```python
from build123d import *

# Parameters (mm, degrees)
SZKIC1_W                    = 80
SZKIC1_H                    = 80
DODANIE_WYCI_GNI_CIE1_DEPTH = 60
SZKIC2_W                    = 77
SZKIC2_H                    = 57
WYTNIJ_WYCI_GNI_CIE1_DEPTH  = 108.703296143
SZKIC4_R                    = 4
WYTNIJ_WYCI_GNI_CIE2_DEPTH  = 81.305666052
SZKIC3_R                    = 4
WYTNIJ_WYCI_GNI_CIE3_DEPTH  = 60
ZAOKR_GLENIE1_R             = 5
SFAZOWANIE1_SIZE            = 1


with BuildPart() as part:
    # Szkic1 → Dodanie-wyciągnięcie1 (new body)
    with BuildSketch(Plane(origin=(0, 0, 0), x_dir=(1, 0, 0), z_dir=(0, 1, 0))):
        Rectangle(SZKIC1_W, SZKIC1_H)
    extrude(amount=DODANIE_WYCI_GNI_CIE1_DEPTH)

    # Szkic2 → Wytnij-wyciągnięcie1 (cut, through all)
    with BuildSketch(Plane.XY.offset(40)):
        with Locations((1.5, 31.5)):
            Rectangle(SZKIC2_W, SZKIC2_H)
    extrude(amount=-WYTNIJ_WYCI_GNI_CIE1_DEPTH, mode=Mode.SUBTRACT)

    # Szkic4 → Wytnij-wyciągnięcie2 (cut, through all)
    with BuildSketch(Plane(origin=(0, 3, 0), x_dir=(1, 0, 0), z_dir=(0, 1, 0))):
        with Locations(Location((20, -20, 0), (0, 0, 180))):
            Circle(SZKIC4_R)
        with Locations(Location((20, 20, 0), (0, 0, 180))):
            Circle(SZKIC4_R)
        with Locations(Location((-20, 20, 0), (0, 0, 180))):
            Circle(SZKIC4_R)
        with Locations((-20, -20)):
            Circle(SZKIC4_R)
    extrude(amount=-WYTNIJ_WYCI_GNI_CIE2_DEPTH, mode=Mode.SUBTRACT)

    # Szkic3 → Wytnij-wyciągnięcie3 (cut)
    with BuildSketch(Plane(origin=(-37, 0, 0), x_dir=(0, 0, -1), z_dir=(1, 0, 0))):
        with Locations(Location((-20, 46.5, 0), (0, 0, 90))):
            Circle(SZKIC3_R)
        with Locations((-20, 16.5)):
            Circle(SZKIC3_R)
        with Locations(Location((20, 16.5, 0), (0, 0, 90))):
            Circle(SZKIC3_R)
        with Locations((20, 46.5)):
            Circle(SZKIC3_R)
    extrude(amount=-WYTNIJ_WYCI_GNI_CIE3_DEPTH, mode=Mode.SUBTRACT)

    # Zaokrąglenie1
    zaokr_glenie1_edges = [part.edges().sort_by_distance(p)[0] for p in [
        (-38.5, 60, -40),
        (40, 1.5, 40),
        (40, 1.5, -40),
        (-38.5, 60, 40),
    ]]
    fillet(zaokr_glenie1_edges, radius=ZAOKR_GLENIE1_R)

    # Sfazowanie1
    sfazowanie1_edges = [part.edges().sort_by_distance(p)[0] for p in [
        (-24, 3, 20),
        (-24, 0, 20),
        (-16, 0, -20),
        (-16, 3, -20),
        (24, 3, -20),
        (24, 0, -20),
        (24, 0, 20),
        (24, 3, 20),
        (-40, 46.5, -16),
        (-37, 46.5, -16),
        (-40, 12.5, -20),
        (-37, 12.5, -20),
        (-40, 16.5, 24),
        (-37, 16.5, 24),
        (-40, 42.5, 20),
        (-37, 42.5, 20),
    ]]
    chamfer(sfazowanie1_edges, length=SFAZOWANIE1_SIZE)


solid = part.part
```
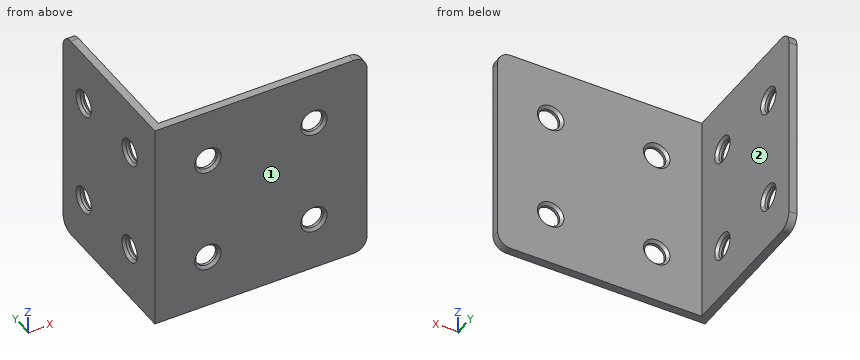
CAD build for the part. Positions are in the model's coordinates, mm. Face numbers are marked on the shaded views. A direction names the side the tool comes from. Give positions to 0.01 mm unless a question says otherwise; leave off trailing zeros. Write each loop counter-clockwise with the first axis right and the second up, starting at its lowest first coordinate (ties: lowest second). Pieces come first, ordered by that corner, then holes. Notation, with made-up numbers: M 17,-5 L 61,-5 A27 cw 61,33 Z; hole C 13.25,14.25 d10. An arc over 180 degrees is marked long. Return JSON: item names as keys, results as strings. Group by question number.
(1) Band-saw the part on C-C (z = 20). State how many separate pieces and enclosed holes the cut face has, and give its area (3 significant figures).
(2) 3-axis set-ups, long thin cutter, end or side, ignore diameter. For the marked faces 1 and 2: which of +Z, -Z, +X, -X, +Y, -Y reach the whole face in a straight line?
(3) Band-saw the part on A-A (x = -20). Give the cut face in (y, z), and give its area (3 significant figures).
(4) Drill centre lines: L1, parallel to Z at x = -20, y = 1.45; L2, parallel to X at y = 14.5, z = -25; L3, parallel to Y at x = -26, z = 31. Where is each one in solid material? Low to high. Write a range as [from, to].
(5) Band-saw the part on B-B (y = 16.5). Give the cut face in (x, z), and give its area (3 significant figures).
(6) Flat gauge pins, fed straight in: pin 1 Ø1.5 at (x, z) = (-4.5, -11.5) entering from +Y; pin 2 Ø10.5 at (y, z) = (46.5, 20) entering from +X. Where does each tip first touch, or does it go through?
(7) Band-saw the part on D-D (z = -6). Give the cut face in (x, y), and give its area (3 significant figures).
Entries:
{
 "1": {"separate pieces": "5", "enclosed holes": "0", "area": "307 mm^2"},
 "2": {"face 1": "+Z, -Z, +X, -X, -Y", "face 2": "+Z, -Z, +X, +Y"},
 "3": {"outline": "M 0,-40 L 3,-40 L 3,-25 L 2,-24 L 1,-24 L 0,-25 Z; M 0,-15 L 1,-16 L 2,-16 L 3,-15 L 3,15 L 2,16 L 1,16 L 0,15 Z; M 0,25 L 1,24 L 2,24 L 3,25 L 3,40 L 0,40 Z", "area": "188 mm^2"},
 "4": {"L1": "z = [-40, -24], [-16, 16], [24, 40]", "L2": "x = [-40, -37]", "L3": "y = [0, 3]"},
 "5": {"outline": "M -40,-40 L -37,-40 L -37,-25 L -38,-24 L -39,-24 L -40,-25 Z; M -40,-15 L -39,-16 L -38,-16 L -37,-15 L -37,15 L -38,16 L -39,16 L -40,15 Z; M -40,25 L -39,24 L -38,24 L -37,25 L -37,40 L -40,40 Z", "area": "188 mm^2"},
 "6": {"pin 1": "stops at y = 3", "pin 2": "stops at x = -37"},
 "7": {"outline": "M -40,0 L 40,0 L 40,3 L -37,3 L -37,60 L -40,60 Z", "area": "411 mm^2"}
}
